```python
from build123d import *

# Parameters (mm, degrees)
SKETCH_W        = 27
SKETCH_H        = 27
PAD_DEPTH       = 4.6
SKETCH001_W     = 20.2
SKETCH001_H     = 24.4
POCKET_DEPTH    = 2
SKETCH002_W     = 16.4
SKETCH002_H     = 3
POCKET001_DEPTH = 2
CHAMFER_SIZE    = 1
SKETCH003_R     = 2
POCKET002_DEPTH = 4.601


with BuildPart() as part:
    # Sketch → Pad (new body)
    with BuildSketch(Plane.XY):
        Rectangle(SKETCH_W, SKETCH_H)
    extrude(amount=PAD_DEPTH)

    # Sketch001 (on Face6 of Pad) → Pocket (cut)
    with BuildSketch(Plane.XY.offset(4.6)):
        Rectangle(SKETCH001_W, SKETCH001_H)
    extrude(amount=-POCKET_DEPTH, mode=Mode.SUBTRACT)

    # Sketch002 (on Face11 of Pocket) → Pocket001 (cut)
    with BuildSketch(Plane.XY.offset(2.6)):
        with Locations((0, 6.2)):
            Rectangle(SKETCH002_W, SKETCH002_H)
    extrude(amount=-POCKET001_DEPTH, mode=Mode.SUBTRACT)

    # Chamfer
    chamfer_edges = [part.edges().sort_by_distance(p)[0] for p in [
        (0, 7.7, 2.6),
        (-8.2, 6.2, 2.6),
        (0, 4.7, 2.6),
        (8.2, 6.2, 2.6),
    ]]
    chamfer(chamfer_edges, length=CHAMFER_SIZE)

    # Sketch003 (on Face14 of Chamfer) → Pocket002 (cut, through all)
    with BuildSketch(Plane.XY.offset(4.6)):
        with Locations((-10.1, 0.5)):
            Circle(SKETCH003_R)
        with Locations((10.1, 0.5)):
            Circle(SKETCH003_R)
    extrude(amount=-POCKET002_DEPTH, mode=Mode.SUBTRACT)


solid = part.part
```
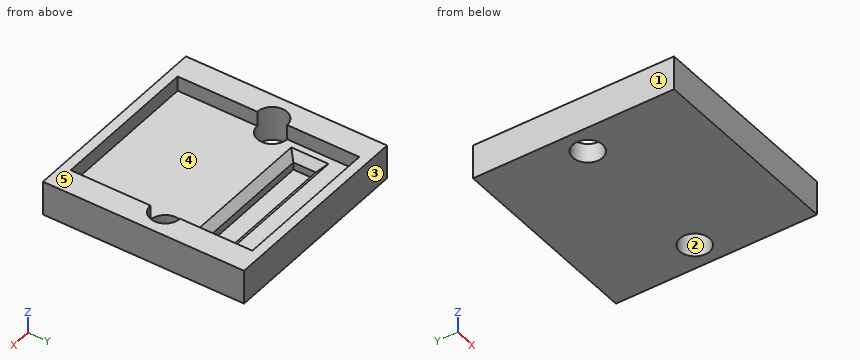
Verification items for the finished model (mm, model axes). Face numbers are marked on the shaded views. A direction names the side the tool comes from. Round coordinates to 2 decimals unless told otherwise and drop trailing zeros. Write each loop counter-clockwise with the first axis right and the second up, starting at its lowest first coordinate (ties: lowest second). Pieces come first, ordered by that corner, then holes. Notation, with made-up numbers: (4.25, 66.25) - (43.25, 66.25) arc R15 ccw to (43.25, 92.25) - close; hole circle Ø3 at (49, -18.75). An arc over 180 degrees is marked (long way). Answer as a JSON object with one key per item and string values. Group by question number.
Q1. Go/stop test with flat-tipped pins: pin 1 Ø3 at (x, y) = (10.1, 0.5) entering from -Z; pin 2 Ø3.5 at (x, y) = (3, 6) entering from +Z. Record where each tip stops, or that it passes through.
Q2. Section check B-B, the plane z = 2.1. Enter the section's corners in (x, y), plus the area to 3 significant figures.
Q3. Section check C-C, the plane z = 3.8. Enter the section's corners in (x, y).
Q4. Section check A-A, the plane y = 0.5. Enter the section's corners in (x, z).
Q5. Section check D-D, the plane x = 0.5. Enter the section's corners in (y, z), plus the area to 3 significant figures.
Q6. Mould release check, pull along Y, two halves, no side actions. Record for the marked faces 1, 2 and 3: released by +Y, released by -Y, zero draft, split by the parting line, or undercut.
Q7. Tool access check on the marked faces 4 and 5. Record the directions out of +Z, -Z, +X, -X, +Y, -Y that give a thin tool (end or side, any length) a straight path to the whole face; none if there is none.
Q8. Thickness scan on line 1 (Y direction, x = 7.75, z = 3.95); line 2 (X direction, y = 0.5, z = 1.65); line 3 (X direction, y = -3.25, z = 2.7). Record the ranges inside material, lowest first.
Found:
{
 "1": {"pin 1": "passes through", "pin 2": "stops at z = 2.05"},
 "2": {"outline": "(-13.5, -13.5) - (13.5, -13.5) - (13.5, 13.5) - (-13.5, 13.5) - close; hole circle Ø4 at (-10.1, 0.5); hole (-8.7, 4.2) - (8.7, 4.2) - (8.7, 8.2) - (-8.7, 8.2) - close; hole circle Ø4 at (10.1, 0.5)", "area": "634 mm^2"},
 "3": {"outline": "(-13.5, -13.5) - (13.5, -13.5) - (13.5, 13.5) - (-13.5, 13.5) - close; hole (-10.1, -12.2) - (10.1, -12.2) - (10.1, -1.5) arc R2 ccw to (10.1, 2.5) - (10.1, 12.2) - (-10.1, 12.2) - (-10.1, 2.5) arc R2 ccw to (-10.1, -1.5) - close"},
 "4": {"outline": "(-13.5, 0) - (-12.1, 0) - (-12.1, 4.6) - (-13.5, 4.6) - close; (-8.1, 0) - (8.1, 0) - (8.1, 2.6) - (-8.1, 2.6) - close; (12.1, 0) - (13.5, 0) - (13.5, 4.6) - (12.1, 4.6) - close"},
 "5": {"outline": "(-13.5, 0) - (13.5, 0) - (13.5, 4.6) - (12.2, 4.6) - (12.2, 2.6) - (8.7, 2.6) - (7.7, 1.6) - (7.7, 0.6) - (4.7, 0.6) - (4.7, 1.6) - (3.7, 2.6) - (-12.2, 2.6) - (-12.2, 4.6) - (-13.5, 4.6) - close", "area": "68.4 mm^2"},
 "6": {"face 1": "zero draft", "face 2": "undercut", "face 3": "released by +Y"},
 "7": {"face 4": "+Z", "face 5": "+Z, +X, -X, +Y, -Y"},
 "8": {"line 1": "y = -13.5 to -12.2, 12.2 to 13.5", "line 2": "x = -13.5 to -12.1, -8.1 to 8.1, 12.1 to 13.5", "line 3": "x = -13.5 to -10.1, 10.1 to 13.5"}
}
